The drawing under review shows one solid part. Ordinate dimensions are in mm from its lowest x, y, z. Coordinates: 2 decimals unless noted, no trailing zeros. Order: outer loops, then holes, each group sorted by start corner. A loop starts at its lowest first (then second) coordinate and runs counter-clockwise, first axis right, second up.
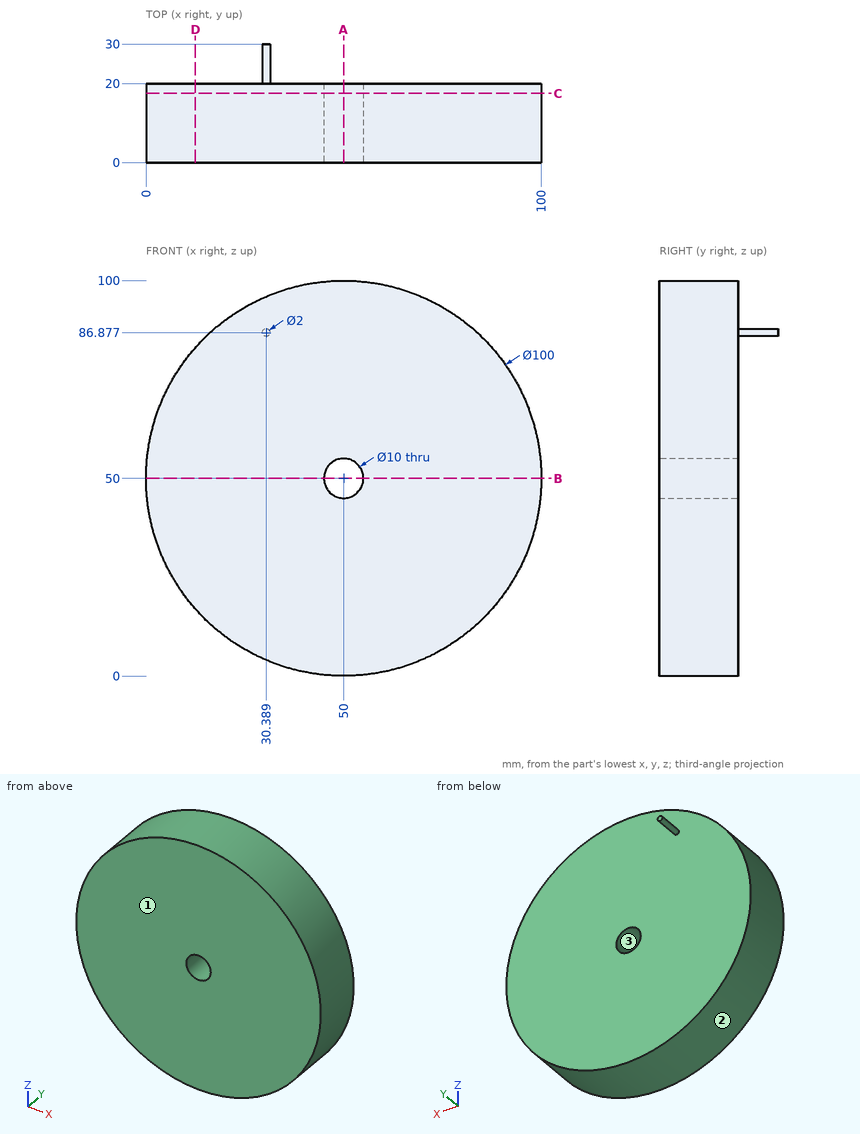
1. To check wall thickness, follow L1, parallel to X at y = 12, z = 50; L2, parallel to Y at x = 20.5, z = 32.5; L3, parallel to Z at x = 8, y = 5. State the ranges of each line that lie inside material, in increasing order.
Answer below:
L1: x = 0 to 45, 55 to 100
L2: y = 0 to 20
L3: z = 22.87 to 77.13
2. Take a section at B-B, the plane z = 50. Give the boundary of the cut face in (x, y), plus the area to 3 significant figures.
Answer below:
outline: (0, 0) - (45, 0) - (45, 20) - (0, 20) - close; (55, 0) - (100, 0) - (100, 20) - (55, 20) - close
area: 1,800 mm2
3. The part is to be moulded in two halves that separate along Z. For the marked faces 1, 2 and 3, say which applies: +Z half, -Z half, draft (parallel to the pull), parting line (faces both ways), or undercut.
Answer below:
face 1: draft
face 2: parting line
face 3: undercut
4. Clearance check with flat-ended pins moving along their axes: pin 1 Ø1 at (x, y) = (88, 10) entering from -Z; pin 2 Ø5 at (y, z) = (5, 63.5) entering from -X (1 decimal); pin 3 Ø1.5 at (x, z) = (13, 40.5) entering from +Y. State where each tip first meets the part, or that it passes through.
Answer below:
pin 1: stops at z = 16.93
pin 2: stops at x = 1.2
pin 3: stops at y = 20
5. Take a section at D-D, the plane x = 12.5. Give the boundary of the cut face in (y, z).
Answer below:
outline: (0, 16.93) - (20, 16.93) - (20, 83.07) - (0, 83.07) - close
6. Take a section at C-C, the plane y = 17.5. Give the boundary of the cut face in (x, z), plus the area to 3 significant figures.
Answer below:
outline: circle Ø100 at (50, 50); hole circle Ø10 at (50, 50)
area: 7,780 mm2
7. Take a section at A-A, the plane x = 50. Give the boundary of the cut face in (y, z), plus the area to 3 significant figures.
Answer below:
outline: (0, 0) - (20, 0) - (20, 45) - (0, 45) - close; (0, 55) - (20, 55) - (20, 100) - (0, 100) - close
area: 1,800 mm2
